from build123d import *

# Parameters (mm, degrees)
BOSS_EXTRU_1_DEPTH      = 113.7
BOSS_EXTRU_2_DEPTH      = 10
ENL_V_MAT_EXTRU_1_DEPTH = 10
ESQUISSE7_R             = 2.135429921
BOSS_EXTRU_3_DEPTH      = 8


with BuildPart() as part:
    # Esquisse1 → Boss.-Extru.1 (new body)
    with BuildSketch(Plane(origin=(0, 0, 0), x_dir=(0, 0, -1), z_dir=(1, 0, 0))):
        Polygon((0.098261178, 46.06547401), (5.004980628, 45.792878485), (0.068148881, -43.07009295), (-4.838570569, -42.797497425), align=None)
    extrude(amount=BOSS_EXTRU_1_DEPTH)

    # Esquisse4 → Boss.-Extru.2 (add, symmetric)
    with BuildSketch(Plane.ZY):
        Polygon((-5.004980628, 45.792878485), (-6.904980628, 45.792878485), (-1.968148881, -43.175523419), (-0.068148881, -43.07009295), align=None)
    boss_extru_2 = extrude(amount=BOSS_EXTRU_2_DEPTH, both=True)

    # Esquisse5 → Enlèv. mat.-Extru.1 (cut)
    with BuildSketch(Plane(origin=(0, -0.241410847, -4.350550784), x_dir=(-1, 0, 0), z_dir=(0, -0.05540448773291252, -0.9984639917087915))):
        with BuildLine():
            Line((3.4, -29.138054447), (3.4, 32.243000428))
            ThreePointArc((3.4, 32.243000428), (5, 33.843000428), (6.6, 32.243000428))
            Line((6.6, 32.243000428), (6.6, -29.138054447))
            ThreePointArc((6.6, -29.138054447), (5, -30.738054447), (3.4, -29.138054447))
        make_face()
    enl_v_mat_extru_1 = extrude(amount=-ENL_V_MAT_EXTRU_1_DEPTH, mode=Mode.SUBTRACT)

    # Esquisse7 → Boss.-Extru.3 (add)
    with BuildSketch(Plane(origin=(0, 0.136297763, 2.453359725), x_dir=(1, 0, 0), z_dir=(0, 0.0554700196225224, 0.9984603532054125))):
        with Locations(Location((56.8495, 25.234545409, 0), (0, 0, 90))):
            Circle(ESQUISSE7_R)
    extrude(amount=BOSS_EXTRU_3_DEPTH)

    # Esquisse8 → Révolution4 (revolve)
    with BuildSketch(Plane(origin=(56.85, 0, 0), x_dir=(0, 0, -1), z_dir=(1, 0, 0))):
        with BuildLine():
            Line((-6.406620571, 29.309512271), (-7.063469335, 22.166281969))
            ThreePointArc((-7.063469335, 22.166281969), (-10.306660104, 26.066321502), (-6.406620571, 29.309512271))
        make_face()
    revolve(axis=Axis((56.85, 29.309512271, 6.406620571), (0, -0.9957988523704411, 0.09156771056279951)))

    # Symétrie1: Boss.-Extru.2, Enlèv. mat.-Extru.1 across plane
    add(boss_extru_2.mirror(Plane(origin=(56.85, 0, 0), x_dir=(0, 0, 1), z_dir=(1, 0, 0))))
    add(enl_v_mat_extru_1.mirror(Plane(origin=(56.85, 0, 0), x_dir=(0, 0, 1), z_dir=(1, 0, 0))), mode=Mode.SUBTRACT)


solid = part.part
Verification items for the finished model (mm, model axes). A direction names the side the tool comes from. Give positions to 0.01 mm unless a question says otherwise; leave off trailing zeros. Write each loop counter-clockwise with the first axis right and the second up, starting at its lowest first coordinate (ties: lowest second). Pieces come first, ordered by that corner, then holes. Notation, with made-up numbers: (17, 66) -> (24, 66) arc R18 ccw to (24, 96) -> close; hole circle Ø6 at (7, 11). An arc over 180 degrees is marked (long way). Use CSV: the item, a comma, the result in double quotes.
(1) Set-up check for faces 1 (the flat face through (120.3, 2, -4)), 2 (the flat face through (113.7, 2, 0)), 3 (the flat face through (-7.3, 0.7, -2.5)): record each of +Z, -Z, +X, -X, +Y, -Y from which the full face is reachable in a straight line by a thin tool's end or side.
Derived:
face 1,"+Z, -Z"
face 2,"+Z, +X, +Y"
face 3,"+Z, -X, +Y"
(2) Sectioned sample at A-A (y = 15). Record the cut outline in (x, z).
Derived:
outline,"(-10, -5.2) -> (-6.6, -5.2) -> (-6.6, -3.29) -> (-10, -3.29) -> close; (-3.4, -5.2) -> (10, -5.2) -> (10, -3.29) -> (103.7, -3.29) -> (103.7, -5.2) -> (117.1, -5.2) -> (117.1, -3.29) -> (113.7, -3.29) -> (113.7, 1.63) -> (0, 1.63) -> (0, -3.29) -> (-3.4, -3.29) -> close; (120.3, -5.2) -> (123.7, -5.2) -> (123.7, -3.29) -> (120.3, -3.29) -> close"
(3) Sectioned sample at D-D (y = 4.5). Record the cut outline in (x, z).
Derived:
outline,"(-10, -4.61) -> (-6.6, -4.61) -> (-6.6, -2.71) -> (-10, -2.71) -> close; (-3.4, -4.61) -> (10, -4.61) -> (10, -2.71) -> (103.7, -2.71) -> (103.7, -4.61) -> (117.1, -4.61) -> (117.1, -2.71) -> (113.7, -2.71) -> (113.7, 2.21) -> (0, 2.21) -> (0, -2.71) -> (-3.4, -2.71) -> close; (120.3, -4.61) -> (123.7, -4.61) -> (123.7, -2.71) -> (120.3, -2.71) -> close"
(4) Go/stop test with flat-tipped pins: pin 1 (2 mm diameter, centred on x = 107.5, y = -18, fed in from -Z); pin 2 (2 mm diameter, centred on y = -29.5, z = 1, fed in from +X); pin 3 (1 mm diameter, centred on x = 93.5, y = -8, fed in from -Z). Record where each tip stops, or that it passes through.
Derived:
pin 1,"stops at z = -3.42"
pin 2,"stops at x = 113.7"
pin 3,"stops at z = -2.04"
(5) Sectioned sample at B-B (x = 7). Record the cut outline in (y, z), plus the area to 3 significant figures.
Derived:
outline,"(-43.18, -1.97) -> (45.79, -6.9) -> (45.79, -5) -> (46.07, -0.1) -> (-42.8, 4.84) -> (-43.07, -0.07) -> close"
area,"607 mm^2"
(6) Release check for a two-part mould opening along X. For faces 4 (the cylindrical face through (58.934, 24.949, 2.498)), 5 (the flat face through (56.054, 1.012, 2.405)), 6 (the flat face through (-3.4, 1, -3)) record: +X half, -X half, draft (parallel to the pull), parting line (faces both ways), or undercut.
Derived:
face 4,"parting line"
face 5,"draft"
face 6,"undercut"
(7) Sectioned sample at C-C (y = -38). Record the cut outline in (x, z).
Derived:
outline,"(-10, -2.26) -> (10, -2.26) -> (10, -0.35) -> (103.7, -0.35) -> (103.7, -2.26) -> (123.7, -2.26) -> (123.7, -0.35) -> (113.7, -0.35) -> (113.7, 4.57) -> (0, 4.57) -> (0, -0.35) -> (-10, -0.35) -> close"
(8) Material ranges on L1, parallel to X at y = -26, z = -2.75; L2, parallel to X at y = 31, z = -3.75; L3, parallel to Y at x = 107, z = -0.5, recorded low to high.
Derived:
L1,"x = -10 to -6.6, -3.4 to 10, 103.7 to 117.1, 120.3 to 123.7"
L2,"x = 0 to 113.7"
L3,"y = -43.09 to 46.04"
